Build history of the part. All positions in model axes, mm. Face numbers are marked on the shaded views. A direction names the side the tool comes from. Round coordinates to 2 decimals unless told otherwise and drop trailing zeros. Write each loop counter-clockwise with the first axis right and the second up, starting at its lowest first coordinate (ties: lowest second). Pieces come first, ordered by that corner, then holes. Notation, with made-up numbers: M 3.5,47.25 L 12.5,47.25 A29 ccw 12.5,77.25 Z; hole C 19,-16.75 d8. An arc over 180 degrees is marked long. Use a Markdown table: item, result.
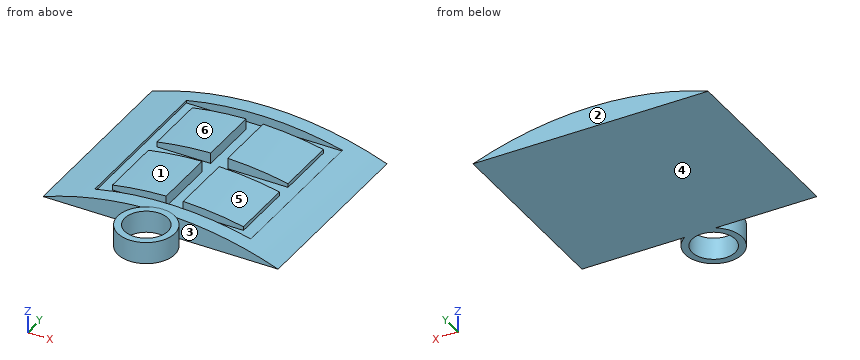
from build123d import *

# Parameters (mm, degrees)
F1_DEPTH      = 12.7
F1_DEPTH_BACK = 12.7
F2_R          = 3.7590001639
F2_R_2        = 2.8460000729
F3_DEPTH      = 2.888742
F5_START      = 1.36109
F4_W          = 20.5638939515
F4_H          = 21.3759541512
F4_W_2        = 2.247471828
F4_H_2        = 8.3905622596
F4_H_3        = 8.2407301525
F4_W_3        = 7.9414884094
F4_H_4        = 1.9977528136
F4_W_4        = 7.082369877
F5_DEPTH      = 1.68691


with BuildPart() as f1:
    # F0 (on Front) → F1 (new body, two sides)
    with BuildSketch(Plane.XZ) as f1_sk:
        with BuildLine():
            ThreePointArc((0, 2.8072327841), (-7.8279825435, 2.0919570377), (-15.405095836, 0))
            Line((-15.405095836, 0), (0, 0))
            Line((0, 0), (0, 2.8072327841))
        make_face()
        with BuildLine():
            Line((0, 2.8072327841), (0, 0))
            Line((0, 0), (15.581065618, 0))
            ThreePointArc((15.581065618, 0), (7.9173771666, 2.1076443124), (0, 2.8072327841))
        make_face()
    extrude(amount=F1_DEPTH)
    extrude(f1_sk.sketch, amount=-F1_DEPTH_BACK)

    # F2 (on Top) → F3 (join)
    with BuildSketch(Plane.XY):
        with Locations((0, -15.8657003194)):
            Circle(F2_R)
        with Locations((0, -15.8657003194)):
            Circle(F2_R_2, mode=Mode.SUBTRACT)
    extrude(amount=F3_DEPTH)

    # F4 (on Top) → F5 (cut)
    with BuildSketch(Plane.XY.offset(F5_START)):
        with Locations((0.5664420314, 0)):
            Rectangle(F4_W, F4_H)
        Polygon((-8.1206136383, 0.9988764068), (-8.1206136383, 9.2396065593), (-1.0382437613, 9.2396065593), (1.2092280667, 9.2396065593), (9.1507164761, 9.2396065593), (9.1507164761, 0.9988764068), (9.1507164761, -0.9988764068), (9.1507164761, -9.3894386664), (1.2092280667, -9.3894386664), (-1.0382437613, -9.3894386664), (-8.1206136383, -9.3894386664), (-8.1206136383, -0.9988764068), align=None, mode=Mode.SUBTRACT)
        with Locations((0.0854921527, -5.1941575366)):
            Rectangle(F4_W_2, F4_H_2)
        with Locations((0.0854921527, 5.119241483)):
            Rectangle(F4_W_2, F4_H_3)
        with Locations((5.1799722714, 0)):
            Rectangle(F4_W_3, F4_H_4)
        with Locations((-4.5794286998, 0)):
            Rectangle(F4_W_4, F4_H_4)
        with Locations((0.0854921527, 0)):
            Rectangle(F4_W_2, F4_H_4)
    extrude(amount=F5_DEPTH, mode=Mode.SUBTRACT)


solid = f1.part
Q1. Cut at B-B on x = 0. Give the cut face in (y, z), and give its area (3 significant figures).
Response values:
| item | result |
|---|---|
| outline | M -19.62,0 L -18.71,0 L -18.71,2.89 L -19.62,2.89 Z; M -13.02,0 L 12.7,0 L 12.7,2.81 L 10.69,2.81 L 10.69,1.36 L -10.69,1.36 L -10.69,2.81 L -12.11,2.81 L -12.11,2.89 L -13.02,2.89 Z |
| area | 44.0 mm2 |
Q2. Which spindle directions (+Z, -Z, +X, -X, +Y, -Y) get a long thin tool onto all of the face, cutting with end or side? Do the marked faces 4, 5 and 6. Say none if no direction does.
Response values:
| item | result |
|---|---|
| face 4 | -Z, +X, -X, +Y, -Y |
| face 5 | +Z, +X, +Y |
| face 6 | +Z, -X, +Y |
Q3. Drill centre lines: L1, parallel to Y at x = 7, z = 1.7; L2, parallel to Y at x = -1, z = 1.75; L3, parallel to Y at x = 0, z = 0.65. Where is each one in solid material? Low to high.
Response values:
| item | result |
|---|---|
| L1 | y = -12.7 to -10.69, -9.39 to -1, 1 to 9.24, 10.69 to 12.7 |
| L2 | y = -19.49 to -18.53, -13.2 to -10.69, 10.69 to 12.7 |
| L3 | y = -19.62 to -18.71, -13.02 to 12.7 |
Q4. Two-plate mould, pull along Y, no slides. Class the marked faces 1, 2 and 3: +Y half, -Y half, draft (parallel to the pull), parting line (faces both ways), or undercut.
Response values:
| item | result |
|---|---|
| face 1 | draft |
| face 2 | +Y half |
| face 3 | undercut |
Q5. Drop flat-ended pins along their axis: P1, Ø0.7, axis at y = 5.5, z = 2, coming from the +X side; P2, Ø0.7, axis at x = 3, z = 1.5, coming from the -Y side; P3, Ø1.4, axis at x = -9.5, z = 1.5, coming from the -Y side; P4, Ø7.5, axis at x = 0, y = -15.87, coming from the +Z side. Give the stop position or say it passes through.
Response values:
| item | result |
|---|---|
| P1 | stops at x = 9.15 |
| P2 | stops at y = -18.53 |
| P3 | stops at y = -12.7 |
| P4 | stops at z = 2.89 |
Q6. Cut at D-D on z = 0.85. Give the cut face in (x, y).
Response values:
| item | result |
|---|---|
| outline | M -12.91,-12.7 L -2.03,-12.7 A3.76 ccw long 2.03,-12.7 L 13.09,-12.7 L 13.09,12.7 L -12.91,12.7 Z; hole C 0,-15.87 d5.69 |
Q7. Cut at C-C on y = -13.5. Give the cut face in (x, z).
Response values:
| item | result |
|---|---|
| outline | M -2.92,0 L -1.58,0 L -1.58,2.89 L -2.92,2.89 Z; M 1.58,0 L 2.92,0 L 2.92,2.89 L 1.58,2.89 Z |
Q8. Cut at A-A on y = 2. Give the cut face in (x, z).
Response values:
| item | result |
|---|---|
| outline | M -15.41,0 L 15.58,0 A44.16 ccw 10.85,1.48 L 10.85,1.36 L 9.15,1.36 L 9.15,1.87 A44.16 ccw 1.21,2.79 L 1.21,1.36 L -1.04,1.36 L -1.04,2.79 A44.16 ccw -8.12,2.04 L -8.12,1.36 L -9.72,1.36 L -9.72,1.71 A44.16 ccw Z |
